The figure shows three views and two pictorial views of one solid part (mm, origin at its lowest corner). Answer the questions. A direction names the side the tool comes from. Coordinates: 2 decimals unless noted, no trailing zeros. Order: outer loops, then holes, each group sorted by start corner. A loop starts at its lowest first (then second) coordinate and runs counter-clockwise, first axis right, second up. Notation, with made-up numbers: (-25.5, 15) -> (17.5, 15) arc R20 ccw to (17.5, 48) -> close; hole circle Ø4 at (40.25, -10.75). An arc over 180 degrees is marked (long way). Return JSON: item names as keys, results as strings.
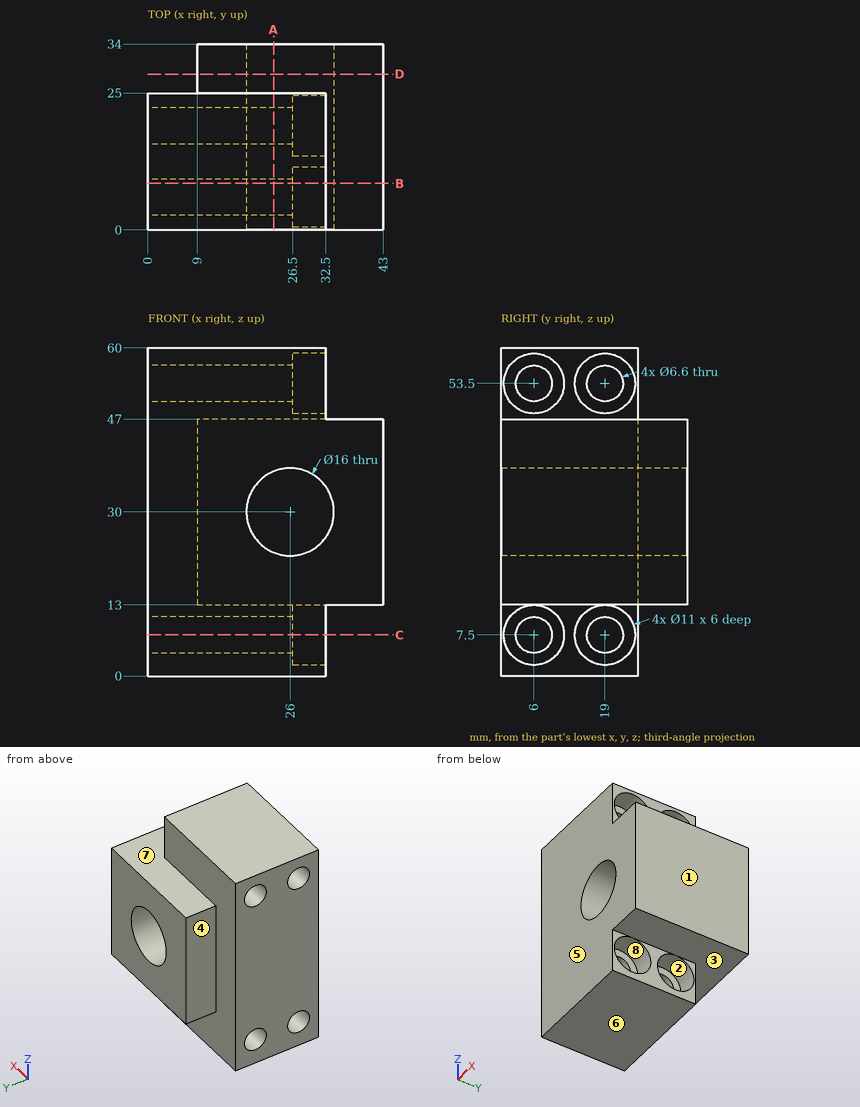
Item 1: Determine the mould class of the marked faces 5, 6, 7 and 8 for opening direction Z: pulls with the +Z half, pulls with the -Z half, needs draft (parallel to the pull), parting line crosses it, or undercut.
Answer list:
{"face 5": "needs draft", "face 6": "pulls with the -Z half", "face 7": "pulls with the +Z half", "face 8": "undercut"}
Item 2: The part is cut by section D-D on y = 28.5. Determine the outline of the cut face in (x, z), plus the area to 3 significant figures.
Answer list:
{"outline": "(9, 13) -> (43, 13) -> (43, 47) -> (9, 47) -> close; hole circle Ø16 at (26, 30)", "area": "955 mm2"}
Item 3: Flat-ended cylindrical pins translate along their axes: pin 1 (9 mm diameter, centred on y = 4.5, z = 10, fed in from +X); pin 2 (5.5 mm diameter, centred on y = 17, z = 9, fed in from +X); pin 3 (12 mm diameter, centred on y = 18.5, z = 56, fed in from +X); pin 4 (4 mm diameter, centred on x = 38.5, y = 24.5, fed in from +Z). Find the tip coordinate at first contact, or state that the pin passes through.
Answer list:
{"pin 1": "x = 43", "pin 2": "x = 26.5", "pin 3": "x = 32.5", "pin 4": "z = 47"}
Item 4: The part is cut by section C-C on z = 7.5. Determine the outline of the cut face in (x, y).
Answer list:
{"outline": "(0, 0) -> (32.5, 0) -> (32.5, 0.5) -> (26.5, 0.5) -> (26.5, 2.7) -> (0, 2.7) -> close; (0, 9.3) -> (26.5, 9.3) -> (26.5, 11.5) -> (32.5, 11.5) -> (32.5, 13.5) -> (26.5, 13.5) -> (26.5, 15.7) -> (0, 15.7) -> close; (0, 22.3) -> (26.5, 22.3) -> (26.5, 24.5) -> (32.5, 24.5) -> (32.5, 25) -> (0, 25) -> close"}
Item 5: Find the intervals of material crossed by probe 1 along Y at (x, z) = (28.75, 53.5); probe 2 along Z at (x, y) = (13.75, 6); probe 3 along X at (y, z) = (18.5, 30), in increasing order.
Answer list:
{"probe 1": "0 to 0.5, 11.5 to 13.5, 24.5 to 25", "probe 2": "0 to 4.2, 10.8 to 50.2, 56.8 to 60", "probe 3": "0 to 18, 34 to 43"}
Item 6: Which of the six approach directions +Z, -Z, +X, -X, +Y, -Y give full straight-line access (tool end or side, diameter ignored) to the marked faces 1, 2, 3 and 4?
Answer list:
{"face 1": "+Z, -Z, +X, +Y, -Y", "face 2": "+X", "face 3": "-Z, +X, +Y", "face 4": "+Z, -Z, -X, +Y"}
Item 7: The part is cut by section B-B on y = 8.5. Determine the outline of the cut face in (x, z).
Answer list:
{"outline": "(0, 0) -> (32.5, 0) -> (32.5, 2.6) -> (26.5, 2.6) -> (26.5, 5.35) -> (0, 5.35) -> close; (0, 9.65) -> (26.5, 9.65) -> (26.5, 12.4) -> (32.5, 12.4) -> (32.5, 13) -> (43, 13) -> (43, 47) -> (32.5, 47) -> (32.5, 48.6) -> (26.5, 48.6) -> (26.5, 51.35) -> (0, 51.35) -> close; (0, 55.65) -> (26.5, 55.65) -> (26.5, 58.4) -> (32.5, 58.4) -> (32.5, 60) -> (0, 60) -> close; hole circle Ø16 at (26, 30)"}
Item 8: The part is cut by section A-A on x = 23. Determine the outline of the cut face in (y, z).
Answer list:
{"outline": "(0, 0) -> (25, 0) -> (25, 13) -> (34, 13) -> (34, 22.58) -> (0, 22.58) -> close; (0, 37.42) -> (34, 37.42) -> (34, 47) -> (25, 47) -> (25, 60) -> (0, 60) -> close; hole circle Ø6.6 at (6, 7.5); hole circle Ø6.6 at (6, 53.5); hole circle Ø6.6 at (19, 7.5); hole circle Ø6.6 at (19, 53.5)"}
